Design review of the part shown in the three views and the two pictorial views. Dimensions are in mm from the part's minimum x, y and z. A direction names the side the tool comes from. Round coordinates to 2 decimals unless told otherwise and drop trailing zeros. Order: outer loops, then holes, each group sorted by start corner. A loop starts at its lowest first (then second) coordinate and runs counter-clockwise, first axis right, second up.
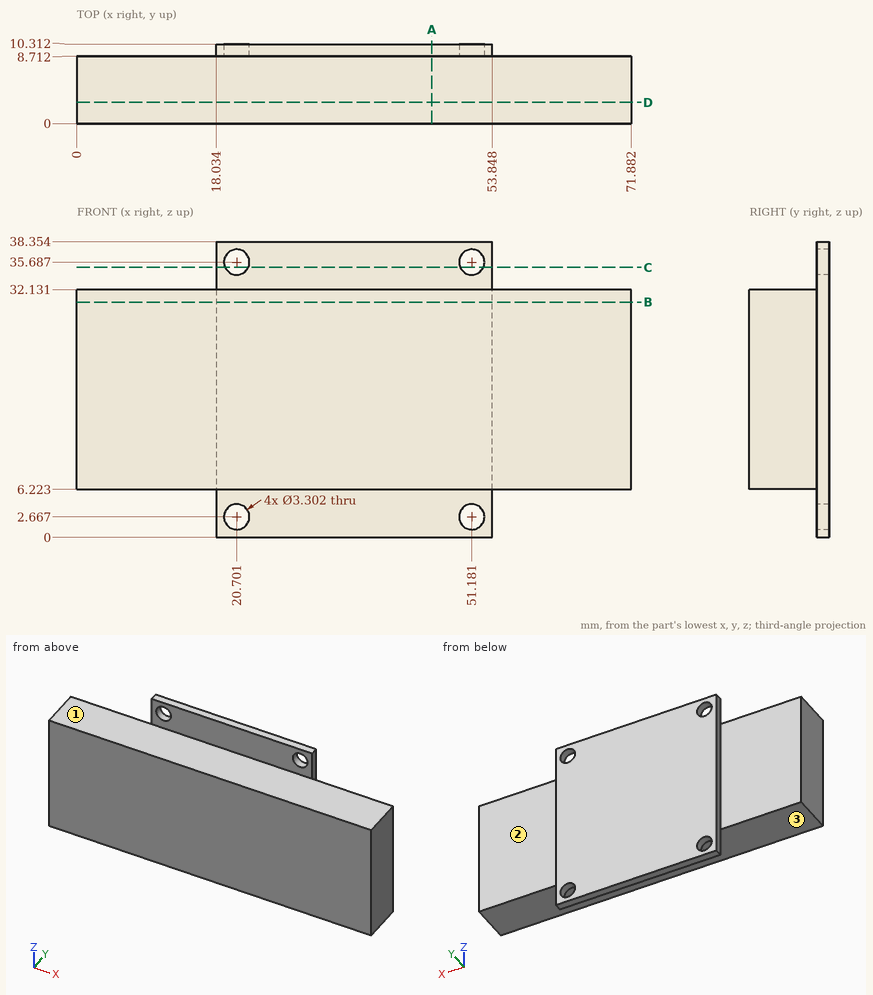
1) To check wall thickness, follow line 1 along Z through (x, y) = (67, 6.5); line 2 along X through (y, z) = (9, 21); line 3 along Y through (x, z) = (14, 13). State the ranges of each line that lie inside material, in increasing order.
Results:
line 1: z = 6.22 to 32.13
line 2: x = 18.03 to 53.85
line 3: y = 0 to 8.71
2) Take a section at B-B on z = 30.5. Give the boundary of the cut face in (x, y).
Results:
outline: (0, 0) - (71.88, 0) - (71.88, 8.71) - (53.85, 8.71) - (53.85, 10.31) - (18.03, 10.31) - (18.03, 8.71) - (0, 8.71) - close
3) Take a section at A-A on x = 46. Give the boundary of the cut face in (y, z), plus the area to 3 significant figures.
Results:
outline: (0, 6.22) - (8.71, 6.22) - (8.71, 0) - (10.31, 0) - (10.31, 38.35) - (8.71, 38.35) - (8.71, 32.13) - (0, 32.13) - close
area: 287 mm2
4) Clearance check with flat-ended pins moving along their axes: P1, Ø1.3, axis at y = 9.5, z = 17, coming from the -X side; P2, Ø6, axis at x = 49.5, y = 8.5, coming from the +Z side; P3, Ø6, axis at x = 15, y = 8, coming from the -Z side; P4, Ø4, axis at x = 20.701, z = 35.687, coming from the -Y side. State where each tip first meets the part, or that it passes through.
Results:
P1: stops at x = 18.03
P2: stops at z = 38.35
P3: stops at z = 6.22
P4: stops at y = 8.71
5) Take a section at D-D on y = 2.75. Give the boundary of the cut face in (x, z), plus the area to 3 significant figures.
Results:
outline: (0, 6.22) - (71.88, 6.22) - (71.88, 32.13) - (0, 32.13) - close
area: 1,860 mm2
6) For the marked faces 1, 2 and 3, list the 3-axis set-ups (+Z, -Z, +X, -X, +Y, -Y) from which the entire face can be reached by the end or side of a thin tool; tool diameter is ignored.
Results:
face 1: +Z, +X, -X, -Y
face 2: +Z, -Z, +X, +Y
face 3: -Z, +X, -X, -Y
7) Take a section at C-C on z = 35. Give the boundary of the cut face in (x, y).
Results:
outline: (18.03, 8.71) - (19.2, 8.71) - (19.2, 10.31) - (18.03, 10.31) - close; (22.2, 8.71) - (49.68, 8.71) - (49.68, 10.31) - (22.2, 10.31) - close; (52.68, 8.71) - (53.85, 8.71) - (53.85, 10.31) - (52.68, 10.31) - close
